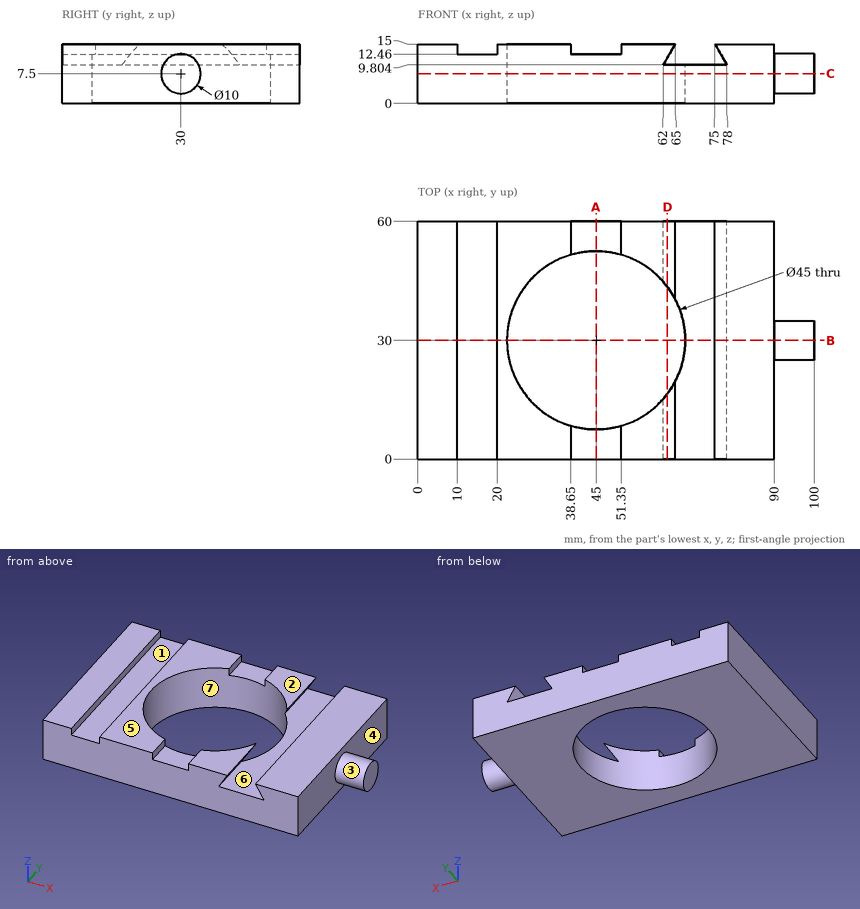
Geometry check sheet. Reference: drawing and pictorial views, mm from the part's lowest x, y, z. A direction names the side the tool comes from. Round coordinates to 2 decimals unless told otherwise and drop trailing zeros. Loops run counter-clockwise (first coordinate to the right, second up) from the corner with the lowest first, then second, coordinate; pieces in that order, holes last. Notation, with made-up numbers: (-8, 62) - (37, 62) arc R19 ccw to (37, 77) - close; hole circle Ø8 at (-13.75, 47). An arc over 180 degrees is marked (long way). Write item = value, one per line. Start each with the question number.
Q1. Section check B-B (y = 30). Record the boundary of the cut face in (x, z), plus the area to 3 significant figures.
Q2. Section check A-A (x = 45). Record the boundary of the cut face in (y, z).
Q3. Section check C-C (z = 7.5). Record the boundary of the cut face in (x, y), plus the area to 3 significant figures.
Q4. Access from +Z, -Z, +X, -X, +Y, -Y to the whole of each face (thin tool, end or side, straight path). Record for the marked faces 1, 2 and 3.
Q5. Depth check by flat-ended pin: P1, Ø1.3, axis at y = 44, z = 14, coming from the +X side; P2, Ø6.5, axis at x = 45.5, y = 54.5, coming from the +Z side; P3, Ø5, axis at x = 70, y = 33, coming from the +Z side. Enter the tip coordinate at first touch or a pass-through.
Q6. Section check D-D (x = 63). Record the boundary of the cut face in (y, z), plus the area to 3 significant figures.
Q7. Release check for a two-part mould opening along X. For the marked faces 4, 5, 6 and 7 record: pulls with the +X half, pulls with the -X half, needs draft (parallel to the pull), parting line crosses it, or undercut.
Q8. Thickness scan on L1, parallel to X at y = 30, z = 7.25; L2, parallel to X at y = 26.5, z = 12.5; L3, parallel to Y at x = 45, z = 5.5. Record the ranges inside material, lowest first.
Derived:
q1.outline = (0, 0) - (22.5, 0) - (22.5, 15) - (20, 15) - (20, 12.46) - (10, 12.46) - (10, 15) - (0, 15) - close; (67.5, 0) - (90, 0) - (90, 2.5) - (100, 2.5) - (100, 12.5) - (90, 12.5) - (90, 15) - (75, 15) - (78, 9.8) - (67.5, 9.8) - close
q1.area = 703 mm^2
q2.outline = (0, 0) - (7.5, 0) - (7.5, 12.46) - (0, 12.46) - close; (52.5, 0) - (60, 0) - (60, 12.46) - (52.5, 12.46) - close
q3.outline = (0, 0) - (90, 0) - (90, 25) - (100, 25) - (100, 35) - (90, 35) - (90, 60) - (0, 60) - close; hole circle Ø45 at (45, 30)
q3.area = 3,910 mm^2
q4.face_1 = +Z, +Y, -Y
q4.face_2 = +Z, +X, -X, +Y, -Y
q4.face_3 = +X
q5.P1 = 90
q5.P2 = 12.46
q5.P3 = 9.8
q6.outline = (0, 0) - (16.5, 0) - (16.5, 9.8) - (0, 9.8) - close; (0, 11.54) - (16.5, 11.54) - (16.5, 15) - (0, 15) - close; (43.5, 0) - (60, 0) - (60, 9.8) - (43.5, 9.8) - close; (43.5, 11.54) - (60, 11.54) - (60, 15) - (43.5, 15) - close
q6.area = 438 mm^2
q7.face_4 = pulls with the +X half
q7.face_5 = needs draft
q7.face_6 = undercut
q7.face_7 = undercut
q8.L1 = 0 to 22.5, 67.5 to 100
q8.L2 = 0 to 10, 20 to 22.77, 76.44 to 90
q8.L3 = 0 to 7.5, 52.5 to 60
